Study the drawing (mm; zero at the part's minimum x, y, z) and answer. A direction names the side the tool comes from. Round coordinates to 2 decimals unless told otherwise and drop trailing zeros. Order: outer loops, then holes, each group sorted by start corner. A loop starts at its lowest first (then second) coordinate and runs counter-clockwise, first axis right, second up. Notation, with made-up numbers: (50.5, 68) -> (70.5, 68) arc R22 cw to (70.5, 91) -> close; hole circle Ø7 at (38.5, 36.5). An arc over 180 degrees is marked (long way). Use one line per item in the form item = value.
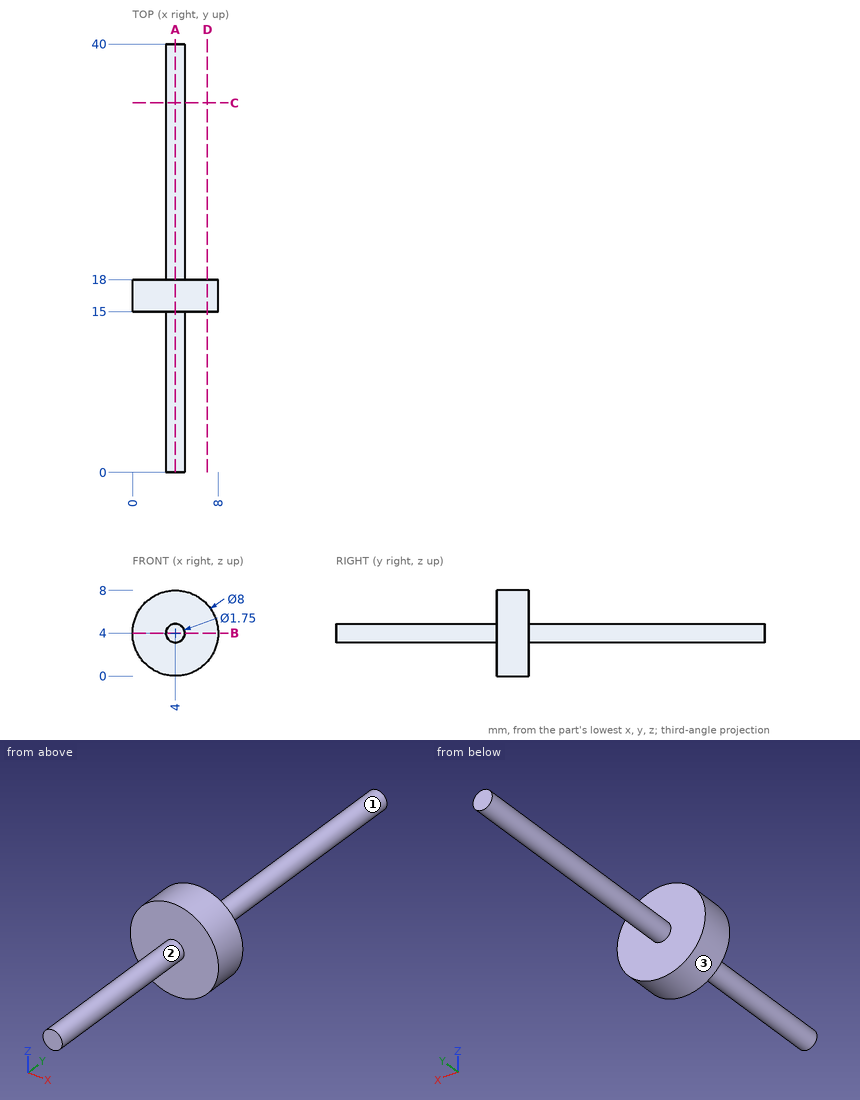
Item 1: The part is cut by section A-A, the plane x = 4. Give the vertices of the cut face in (y, z) (3 decimals).
Findings:
outline = (0, 3.125) -> (15, 3.125) -> (15, 0) -> (18, 0) -> (18, 3.125) -> (40, 3.125) -> (40, 4.875) -> (18, 4.875) -> (18, 8) -> (15, 8) -> (15, 4.875) -> (0, 4.875) -> close
Item 2: The part is cut by section C-C, the plane y = 34.5. Give the vertices of the cut face in (x, z) (3 decimals), and give its area (3 significant figures).
Findings:
outline = circle Ø1.75 at (4, 4)
area = 2.41 mm^2
Item 3: Flat-ended cylindrical pins translate along their axes: P1, Ø3, axis at x = 6, y = 15.5, coming from the -Z side; P2, Ø1.5, axis at y = 28, z = 1.5, coming from the -X side; P3, Ø1, axis at y = 16.5, z = 3.5, coming from the +X side. Find the tip coordinate at first contact, or state that the pin passes through.
Findings:
P1 = 0.03
P2 = through
P3 = 8
Item 4: Consider line 1 along Y through (x, z) = (5, 3); line 2 along X through (y, z) = (4.5, 4) (3 decimals); line 3 along Z through (x, y) = (3.5, 13.5). Determine where each line is inside the solid, lowest interval first.
Findings:
line_1 = 15 to 18
line_2 = 3.125 to 4.875
line_3 = 3.28 to 4.72
Item 5: The part is cut by section D-D, the plane x = 7. Give the vertices of the cut face in (y, z), and give its area (3 significant figures).
Findings:
outline = (15, 1.35) -> (18, 1.35) -> (18, 6.65) -> (15, 6.65) -> close
area = 15.9 mm^2
Item 6: For the marked faces 1, 2 and 3, determine the directions among +Z, -Z, +X, -X, +Y, -Y from which every point of the face is accessible in a straight line to the end or side of a thin tool.
Findings:
face_1 = +Y
face_2 = -Y
face_3 = +Y, -Y
Item 7: The part is cut by section B-B, the plane z = 4. Give the vertices of the cut face in (x, y) (3 decimals).
Findings:
outline = (0, 15) -> (3.125, 15) -> (3.125, 0) -> (4.875, 0) -> (4.875, 15) -> (8, 15) -> (8, 18) -> (4.875, 18) -> (4.875, 40) -> (3.125, 40) -> (3.125, 18) -> (0, 18) -> close
